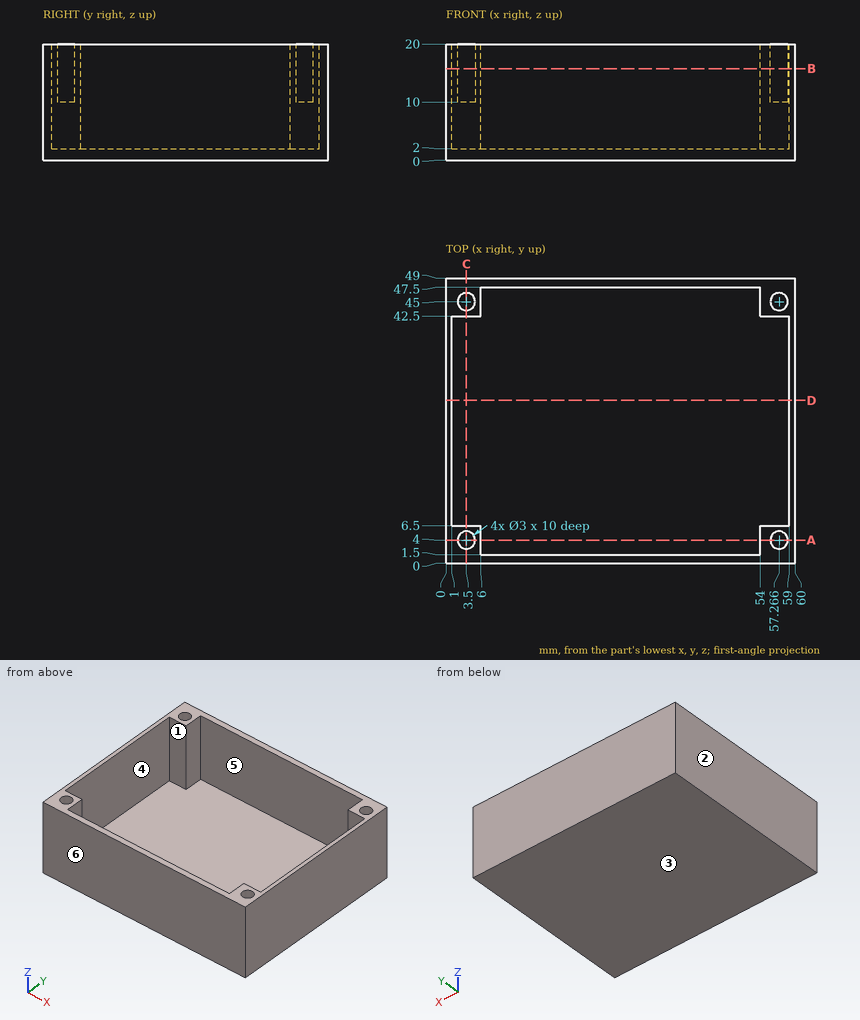
Geometry: see drawing. Coordinates: mm, zero at the bounding-box minimum. A direction names the side the tool comes from. Coordinates: 2 decimals unless noted, no trailing zeros. Loops run counter-clockwise (first coordinate to the right, second up) from the corner with the lowest first, then second, coordinate; pieces in that order, holes last. Notation, with made-up numbers: (32, -37.75) - (36, -37.75) arc R20 ccw to (36, -8.75) - close; hole circle Ø9 at (76.5, 54.25). An arc over 180 degrees is marked (long way). Answer in a Markdown table with one row per item.
(1) Pin query (flat end, axial travel): P1, Ø4, axis at x = 44, y = 17, coming from the -Z side. Return the tip coordinate at first contact, or that it passes through.
Model answer:
| item | result |
|---|---|
| P1 | stops at z = 0 |
(2) Set-up query: the marked faces 1 and 2. Return all of +Z, -Z, +X, -X, +Y, -Y with unobstructed straight access to the full face (end or side cutting, diameter ignored); none if empty.
Model answer:
| item | result |
|---|---|
| face 1 | +Z |
| face 2 | +Z, -Z, -X, +Y, -Y |
(3) Mould query, pull axis Y, two halves, no side actions, for the marked faces 3, 4, 5 and 6. Classes: pulls with the +Y half, pulls with the -Y half, needs draft (parallel to the pull), parting line crosses it, or undercut.
Model answer:
| item | result |
|---|---|
| face 3 | needs draft |
| face 4 | undercut |
| face 5 | undercut |
| face 6 | pulls with the -Y half |
(4) Cut plane B-B on z = 15.75. Output: boundary loops of the cut face in (x, y).
Model answer:
| item | result |
|---|---|
| outline | (0, 0) - (60, 0) - (60, 49) - (0, 49) - close; hole (1, 6.5) - (6, 6.5) - (6, 1.5) - (54, 1.5) - (54, 6.5) - (59, 6.5) - (59, 42.5) - (54, 42.5) - (54, 47.5) - (6, 47.5) - (6, 42.5) - (1, 42.5) - close; hole circle Ø3 at (3.5, 4); hole circle Ø3 at (3.5, 45); hole circle Ø3 at (57.27, 4); hole circle Ø3 at (57.27, 45) |
(5) Cut plane C-C on x = 3.5. Output: boundary loops of the cut face in (y, z).
Model answer:
| item | result |
|---|---|
| outline | (0, 0) - (49, 0) - (49, 20) - (46.5, 20) - (46.5, 10) - (43.5, 10) - (43.5, 20) - (42.5, 20) - (42.5, 2) - (6.5, 2) - (6.5, 20) - (5.5, 20) - (5.5, 10) - (2.5, 10) - (2.5, 20) - (0, 20) - close |
(6) Cut plane D-D on y = 28. Output: boundary loops of the cut face in (x, z), plus the area to 3 significant figures.
Model answer:
| item | result |
|---|---|
| outline | (0, 0) - (60, 0) - (60, 20) - (59, 20) - (59, 2) - (1, 2) - (1, 20) - (0, 20) - close |
| area | 156 mm² |
(7) Material intervals for L1, parallel to Y at x = 3.5, z = 15.25; L2, parallel to X at y = 24, z = 16; L3, parallel to Y at x = 43, z = 3.5, sorted ascending. Write a range as from..to.
Model answer:
| item | result |
|---|---|
| L1 | y = 0..2.5, 5.5..6.5, 42.5..43.5, 46.5..49 |
| L2 | x = 0..1, 59..60 |
| L3 | y = 0..1.5, 47.5..49 |
(8) Cut plane A-A on y = 4. Output: boundary loops of the cut face in (x, z).
Model answer:
| item | result |
|---|---|
| outline | (0, 0) - (60, 0) - (60, 20) - (58.77, 20) - (58.77, 10) - (55.77, 10) - (55.77, 20) - (54, 20) - (54, 2) - (6, 2) - (6, 20) - (5, 20) - (5, 10) - (2, 10) - (2, 20) - (0, 20) - close |
